Geometry check sheet. Reference: the model listing, model coordinates, mm. Face numbers are marked on the shaded views. A direction names the side the tool comes from. Round coordinates to 2 decimals unless told otherwise and drop trailing zeros. Loops run counter-clockwise (first coordinate to the right, second up) from the corner with the lowest first, then second, coordinate; pieces in that order, holes last. Notation, with made-up numbers: (-18.5, 6.25) - (-1.5, 6.25) arc R7 cw to (-1.5, 16.25) - close; hole circle Ø8 at (-39.5, -17.75). An arc over 180 degrees is marked (long way). Answer as CSV lines item,"result". Start each with the question number.
1) Cross-section at C-C on z = -28.5. Record the boundary of the cut face in (x, y), and give its area (3 significant figures).
2) Cross-section at D-D on x = -68. Record the boundary of the cut face in (y, z), and give its area (3 significant figures).
3) Thickness scan on line 1 along X through (y, z) = (-170, -41.5); line 2 along X through (y, z) = (-277, -23.5); line 3 along Y through (x, z) = (21.5, -51). Record the ranges inside material, lowest first.
4) Depth check by flat-ended pin: P1, Ø23, axis at y = -256.5, z = -48, coming from the -X side; P2, Ø12, axis at x = -62, y = -131, coming from the -Z side; P3, Ø2, axis at x = 44.5, z = -46, coming from the +Y side; P4, Ø12, axis at y = -80, z = -56, coming from the -X side. Enter the tip coordinate at first touch or a pass-through.
5) Cross-section at B-B on x = 34.5. Record the boundary of the cut face in (y, z), and give its area (3 significant figures).
6) Access from +Z, -Z, +X, -X, +Y, -Y to the whole of each face (thin tool, end or side, straight path). Record for the marked faces 4, 5, 6 and 7.
7) Draft check along Y on the marked faces 1, 2 and 3. Enter one of: released by +Y, released by -Y, zero draft, split by the parting line, or undercut.
8) Cross-section at A-A on y = -239.5. Record the boundary of the cut face in (x, z), and give its area (3 significant figures).
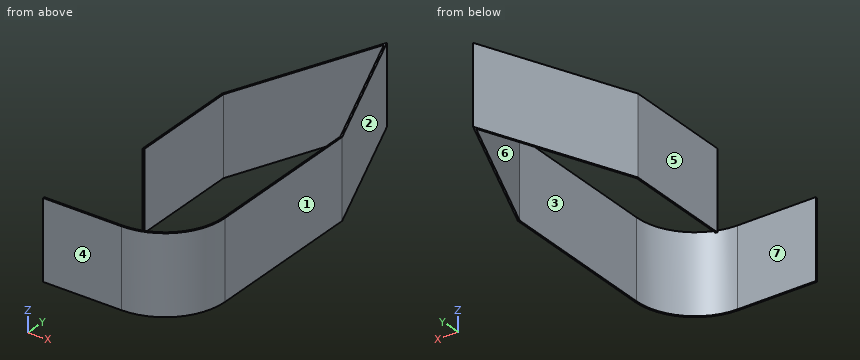
from build123d import *

# Parameters (mm, degrees)
BOSS_EXTRUDE1_DEPTH = 76.2


with BuildPart() as part:
    # Sketch2 → Boss-Extrude1 (new body)
    with BuildSketch(Plane.XY):
        with BuildLine():
            Line((0, 0), (58.320955092, -140.799240755))
            Line((58.320955092, -140.799240755), (58.320955092, -247.213806647))
            Line((58.320955092, -247.213806647), (58.320955092, -298.013806647))
            ThreePointArc((58.320955092, -298.013806647), (41.239142831, -339.252949479), (0, -356.33476174))
            Line((0, -356.33476174), (-76.2, -356.33476174))
            Line((-76.2, -356.33476174), (-76.2, -354.74726174))
            Line((-76.2, -354.74726174), (0, -354.74726174))
            ThreePointArc((0, -354.74726174), (40.116610816, -338.130417463), (56.733455092, -298.013806647))
            Line((56.733455092, -298.013806647), (56.733455092, -247.213806647))
            Line((56.733455092, -247.213806647), (56.733455092, -141.115014138))
            Line((56.733455092, -141.115014138), (0, -4.148337413))
            Line((0, -4.148337413), (-56.733455092, -141.115014138))
            Line((-56.733455092, -141.115014138), (-56.733455092, -247.213806647))
            Line((-56.733455092, -247.213806647), (-58.320955092, -247.213806647))
            Line((-58.320955092, -247.213806647), (-58.320955092, -140.799240755))
            Line((-58.320955092, -140.799240755), (0, 0))
        make_face()
    extrude(amount=-BOSS_EXTRUDE1_DEPTH)


solid = part.part
Answer block:
1,outline,"(-76.2, -356.33) - (0, -356.33) arc R58.32 ccw to (58.32, -298.01) - (58.32, -140.8) - (0, 0) - (-58.32, -140.8) - (-58.32, -247.21) - (-56.73, -247.21) - (-56.73, -141.12) - (0, -4.15) - (56.73, -141.12) - (56.73, -298.01) arc R56.73 cw to (0, -354.75) - (-76.2, -354.75) - close"
1,area,"1,160 mm^2"
2,outline,"(-356.33, -76.2) - (-354.75, -76.2) - (-354.75, 0) - (-356.33, 0) - close"
2,area,"121 mm^2"
3,line 1,"x = -58.32 to -56.73, 56.73 to 58.32"
3,line 2,"x = 56.73 to 58.32"
3,line 3,"y = -352.23 to -350.52, -56.05 to -51.91"
4,P1,"stops at x = -58.32"
4,P2,"passes through"
4,P3,"stops at y = -105.02"
4,P4,"stops at x = -35.62"
5,outline,"(-345.04, -76.2) - (-343.05, -76.2) - (-343.05, 0) - (-345.04, 0) - close; (-87.44, -76.2) - (-83.29, -76.2) - (-83.29, 0) - (-87.44, 0) - close"
5,area,"467 mm^2"
6,face 4,"+Z, -Z, +X, -X, -Y"
6,face 5,"+Z, -Z, -X, +Y"
6,face 6,"+Z, -Z"
6,face 7,"+Z, -Z, -X"
7,face 1,"zero draft"
7,face 2,"released by +Y"
7,face 3,"undercut"
8,outline,"(-58.32, -76.2) - (-56.73, -76.2) - (-56.73, 0) - (-58.32, 0) - close; (56.73, -76.2) - (58.32, -76.2) - (58.32, 0) - (56.73, 0) - close"
8,area,"242 mm^2"
